Build history of the part. All positions in model axes, mm. Round coordinates to 2 decimals unless told otherwise and drop trailing zeros. Write each loop counter-clockwise with the first axis right and the second up, starting at its lowest first coordinate (ties: lowest second). Pieces come first, ordered by that corner, then holes. Notation, with made-up numbers: (25, -17.75) - (76, -17.75) arc R33 ccw to (76, 21.25) - close; hole circle Ø4 at (13, 81.5). An arc over 180 degrees is marked (long way). Answer as a JSON object with one key per item and string values. Group by question number.
Item 1: Probe line 1 (Y direction, x = 1.65, z = -12.7); line 2 (Z direction, x = 2.5, y = -1.5); line 3 (Z direction, x = 2.9, y = 7.5). List the from-to ranges inside material, lowest first. Write a range as from..to.
Item 2: Slice it at A-A, the plane z = -12.7. List the corners of the cut face in (x, y) (3 decimals).
Item 3: Slice it at C-C, the plane x = 2.15. List the corners of the cut face in (y, z).
Item 4: Slice it at B-B, the plane y = 0. List the corners of the cut face in (x, z) (3 decimals), then the cut area to 3 significant figures.
Item 5: Slice it at D-D, the plane y = -6.5. List the corners of the cut face in (x, z) (3 decimals), then the cut area to 3 significant figures.
Item 6: Flat gauge pin, fed straight in: pin 1 (1.5 mm diameter, centred on x = 2, y = 2, fed in from +Z). Where does the tip first touch, or does it go through?
Item 7: Two-plate mould, pull along Z, no slides. Class faces 1 (the cylindrical face through (1.61, -1.673, -10.518)), 2 (the flat face through (2, -12.7, -45)), 3 (the flat face through (2, 0, -88.9)): +Z half, -Z half, draft (parallel to the pull), parting line (faces both ways), or undercut.
Autodesk Inventor part; units mm, degrees
ref_plane "YZ Plane" through (0, 0, 0) normal (1, 0, 0) x (0, 1, 0)
ref_plane "XZ Plane" through (0, 0, 0) normal (0, 1, 0) x (-1, 0, 0)
ref_plane "XY Plane" through (0, 0, 0) normal (0, 0, 1) x (1, 0, 0)
sketch "Sketch1" plane through (0, 0, 0) normal (1, 0, 0) x (0, 1, 0)
  circle A0 centre (0, 0) radius 12.7
  line L0 (0, 12.7) -> (0, -88.9)
  line L1 (12.7, 0) -> (12.7, -88.9)
  line L2 (12.7, -88.9) -> (0, -88.9)
  line L3 (-12.7, -88.9) -> (-12.7, 0)
  line L4 (0, -88.9) -> (-12.7, -88.9)
  dimension "d0" = 25.4
  dimension "d1" = 101.6
extrude "Extrusion1" add sketch "Sketch1" along normal blind 3.175
sketch "Sketch6" plane through (3.175, 0, 0) normal (1, 0, 0) x (0, 0, -1)
  circle A0 centre (12.7, 0) radius 2.75
  point P0 (0, 0)
  dimension "d8" = 5.5
extrude "Extrusion2" cut sketch "Sketch6" against normal through all
properties part number "thing4" material "Aluminum 6061"
Geometry says:
{
 "1": {"line 1": "y = -12.7..-2.75, 2.75..12.7", "line 2": "z = -88.9..-15, -10.4..12.61", "line 3": "z = -88.9..10.25"},
 "2": {"outline": "(0, -12.7) - (3.175, -12.7) - (3.175, -2.75) - (0, -2.75) - close; (0, 2.75) - (3.175, 2.75) - (3.175, 12.7) - (0, 12.7) - close"},
 "3": {"outline": "(-12.7, -88.9) - (12.7, -88.9) - (12.7, 0) arc R12.7 ccw to (-12.7, 0) - close; hole circle Ø5.5 at (0, -12.7)"},
 "4": {"outline": "(0, -88.9) - (3.175, -88.9) - (3.175, -15.45) - (0, -15.45) - close; (0, -9.95) - (3.175, -9.95) - (3.175, 12.7) - (0, 12.7) - close", "area": "305 mm^2"},
 "5": {"outline": "(0, -88.9) - (3.175, -88.9) - (3.175, 10.911) - (0, 10.911) - close", "area": "317 mm^2"},
 "6": {"pin 1": "stops at z = 12.64"},
 "7": {"face 1": "undercut", "face 2": "draft", "face 3": "-Z half"}
}
